Build history of the part. All positions in model axes, mm. Face numbers are marked on the shaded views. Round coordinates to 2 decimals unless told otherwise and drop trailing zeros. Loops run counter-clockwise (first coordinate to the right, second up) from the corner with the lowest first, then second, coordinate; pieces in that order, holes last. Notation, with made-up numbers: (30, 7.5) -> (49, 7.5) arc R21 ccw to (49, 33.5) -> close; hole circle Ø1 at (-23.5, -33). An arc over 180 degrees is marked (long way). Put each result on its own line as item: value. Start each with the question number.
Item 1: Pull direction Y, two halves, no side cores. Call the marked faces 1, 2, 3 and 4: +Y half, -Y half, draft (parallel to the pull), parting line (faces both ways), or undercut.
Item 2: Cut at B-B, the plane x = 9.75. Count the separate pieces of the cut face and the enclosed holes in it, plus the area to 3 significant figures.
Item 3: Cut at D-D, the plane z = 24. List the corners of the cut face in (x, y), plus the area to 3 significant figures.
Item 4: Cut at C-C, the plane y = -53. List the corners of the cut face in (x, z), plus the area to 3 significant figures.
Item 5: Drill centre lines: probe 1 along Y at (x, z) = (7.5, 2); probe 2 along Y at (x, z) = (0.5, -4); probe 3 along Y at (x, z) = (7.5, 78). Where is each one in solid material? Low to high. Write a range as [from, to].
Item 6: Flat gauge pins, fed straight in: pin 1 Ø2 at (x, z) = (11, 25) entering from -Y; pin 2 Ø8.5 at (y, z) = (-154.5, -16.78) entering from +X; pin 3 Ø1.5 at (x, z) = (6.5, 60) entering from +Y; pin 4 Ø1.5 at (x, y) = (9, -51) entering from +Z. Where does each tip first touch, or does it go through?
Item 7: Cut at A-A, the plane y = 19.05. List the corners of the cut face in (x, z), plus the area to 3 significant figures.
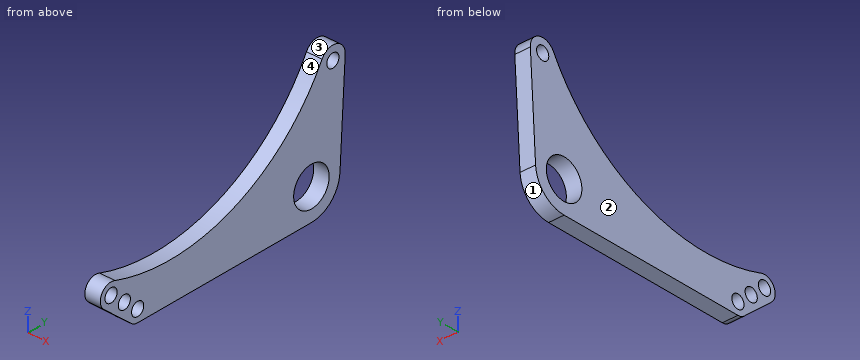
```python
from build123d import *

# Parameters (mm, degrees)
F0_R     = 5.42925
F0_R_2   = 15.8115
F1_DEPTH = 12.7


with BuildPart() as f1:
    # F0 (on Right) → F1 (new body)
    with BuildSketch(Plane.YZ):
        with BuildLine():
            Line((-154.488795, -26.534761), (0, -25.4))
            ThreePointArc((0, -25.4), (17.438947, -18.467353), (25.358361, -1.45379))
            Line((25.358361, -1.45379), (30.010518, 79.693488))
            ThreePointArc((30.010518, 79.693488), (22.077109, 90.874786), (9.422991, 85.59902))
            ThreePointArc((9.422991, 85.59902), (-69.333406, 15.888309), (-174.446099, 12.217438))
            ThreePointArc((-174.446099, 12.217438), (-186.251925, 8.445986), (-184.337166, -3.798813))
            Line((-184.337166, -3.798813), (-160.687818, -24.016462))
            ThreePointArc((-160.687818, -24.016462), (-157.839108, -25.892982), (-154.488795, -26.534761))
        make_face()
        with Locations((-154.498427, -16.776499)):
            Circle(F0_R, mode=Mode.SUBTRACT)
        with Locations((-166.323101, -6.667674)):
            Circle(F0_R, mode=Mode.SUBTRACT)
        with Locations((-178.147775, 3.441151)):
            Circle(F0_R, mode=Mode.SUBTRACT)
        Circle(F0_R_2, mode=Mode.SUBTRACT)
        with Locations((19.05, 80.321853)):
            Circle(F0_R, mode=Mode.SUBTRACT)
    extrude(amount=F1_DEPTH)


solid = f1.part
```
Reply:
1. face 1: +Y half
1. face 2: draft
1. face 3: parting line
1. face 4: undercut
2. separate pieces: 1
2. enclosed holes: 5
2. area: 9,850 mm^2
3. outline: (0, -52.14) -> (12.7, -52.14) -> (12.7, 26.82) -> (0, 26.82) -> close
3. area: 1,000 mm^2
4. outline: (0, -25.79) -> (12.7, -25.79) -> (12.7, 23.53) -> (0, 23.53) -> close
4. area: 626 mm^2
5. probe 1: y = [-187.56, -183.38], [-172.91, -15.68], [15.68, 25.56]
5. probe 2: y = [-184.1, -171.05], [-161.59, -15.3], [15.3, 25.08]
5. probe 3: y = [4.97, 14.14], [23.96, 29.91]
6. pin 1: stops at y = -52.14
6. pin 2: passes through
6. pin 3: stops at y = 28.92
6. pin 4: stops at z = 25.06
7. outline: (0, -16.8) -> (12.7, -16.8) -> (12.7, 74.89) -> (0, 74.89) -> close; (0, 85.75) -> (12.7, 85.75) -> (12.7, 91.3) -> (0, 91.3) -> close
7. area: 1,230 mm^2
